Verification items for the finished model (mm, model axes). A direction names the side the tool comes from. Coordinates: 2 decimals unless noted, no trailing zeros. Loops run counter-clockwise (first coordinate to the right, second up) from the corner with the lowest first, then second, coordinate; pieces in that order, holes last.
Q1. Material ranges on probe 1 along X at (y, z) = (0, 9); probe 2 along Y at (x, z) = (0, -14.95); probe 3 along Z at (x, y) = (0, 13), recorded low to high.
Q2. Mould release check, pull along X, two halves, no side actions. Record for faces 4 (the face through (-0.1, -1.4, 6.6)), 5 (the face through (-2.548, -5.312, 12.573)), 6 (the face through (3, 36, -13.75)), 7 (the face through (-7.707, 29.632, -19.215)): +X half, -X half, draft (parallel to the pull), parting line (faces both ways), or undercut.
Q3. Sectioned sample at D-D (y = 17.5). Enter the section's corners in (x, z).
Q4. Go/stop test with flat-tipped pins: P1, Ø9, axis at y = 8.5, z = -9.5, coming from the +X side; P2, Ø6, axis at x = -6.5, y = 10.5, coming from the +Z side; P3, Ø5, axis at x = 6, z = -2, coming from the -Y side; P4, Ø3, axis at y = 24.5, z = -15.5, coming from the +X side. Record where each tip stops, or that it passes through.
Q5. Sectioned sample at C-C (x = 0). Count the separate pieces of the cut face and the enclosed holes in it, then the cut area to 3 significant figures.
Q6. Access from +Z, -Z, +X, -X, +Y, -Y to the whole of each face (thin tool, end or side, straight path). Record for faces 1 (the face through (0, 26, -16.75)), 2 (the face through (0, 2.5, 5)), 3 (the face through (-7.5, 2.7, -9.7)).
```python
from build123d import *

# Parameters (mm, degrees)
BOSS_EXTRUDE5_DEPTH      = 7.5
BOSS_EXTRUDE5_DEPTH_BACK = 7.5
SKETCH8_W                = 33.5
SKETCH8_H                = 5
SKETCH9_R                = 10
BOSS_EXTRUDE6_DEPTH      = 5
SKETCH11_R               = 2.65
CUT_EXTRUDE7_DEPTH       = 5
SKETCH12_R               = 4
SKETCH12_R_2             = 2.65
BOSS_EXTRUDE7_DEPTH      = 3
CHAMFER1_SIZE            = 3
FILLET1_R                = 10
FILLET2_R                = 5
SKETCH13_R               = 2.65
CUT_EXTRUDE8_DEPTH       = 50
SKETCH14_R               = 4
SKETCH14_R_2             = 2.65
BOSS_EXTRUDE8_DEPTH      = 3
CHAMFER2_SIZE            = 3


with BuildPart() as part:
    # Sketch8 → Boss-Extrude5 (new, two sides: drawn at the far end of the back side and taken through both)
    with BuildSketch(Plane.ZY.offset(-BOSS_EXTRUDE5_DEPTH_BACK)):
        Rectangle(SKETCH8_W, SKETCH8_H)
        Polygon((-16.75, -2.5), (-16.75, 2.5), (-16.75, 41.5), (-21.75, 41.5), (-21.75, -2.5), align=None)
    extrude(amount=BOSS_EXTRUDE5_DEPTH + BOSS_EXTRUDE5_DEPTH_BACK)

    # Sketch9 → Boss-Extrude6 (add)
    with BuildSketch(Plane.XY.offset(-16.75)):
        with Locations((0, 36.5)):
            Circle(SKETCH9_R)
    extrude(amount=-BOSS_EXTRUDE6_DEPTH)

    # Sketch11 → Cut-Extrude7 (cut)
    with BuildSketch(Plane(origin=(0, 0, -21.75), x_dir=(-1, 0, 0), z_dir=(0, 0, -1))):
        with Locations((0, 36.5)):
            Circle(SKETCH11_R)
    extrude(amount=-CUT_EXTRUDE7_DEPTH, mode=Mode.SUBTRACT)

    # Sketch12 → Boss-Extrude7 (add)
    with BuildSketch(Plane.XY.offset(-16.75)):
        with Locations((0, 36.5)):
            Circle(SKETCH12_R)
        with Locations(Location((0, 36.5, 0), (0, 0, 180))):
            Circle(SKETCH12_R_2, mode=Mode.SUBTRACT)
    extrude(amount=BOSS_EXTRUDE7_DEPTH)

    # Chamfer1
    chamfer1_edges = [part.edges().sort_by_distance(p)[0] for p in [
        (-4, 36.5, -16.75),
    ]]
    chamfer(chamfer1_edges, length=CHAMFER1_SIZE - 0.0001)  # a hair under: the kernel refuses the full size

    # Fillet1
    fillet1_edges = [part.edges().sort_by_distance(p)[0] for p in [
        (0, -2.5, -21.75),
        (0, 2.5, -16.75),
    ]]
    fillet(fillet1_edges, radius=FILLET1_R)

    # Fillet2
    fillet2_edges = [part.edges().sort_by_distance(p)[0] for p in [
        (-7.5, 29.885621722, -19.25),
        (7.5, 29.885621722, -19.25),
    ]]
    fillet(fillet2_edges, radius=FILLET2_R)

    # Sketch13 → Cut-Extrude8 (cut)
    with BuildSketch(Plane(origin=(0, 2.5, 0), x_dir=(1, 0, 0), z_dir=(0, 1, 0))):
        with Locations(Location((0, -9.25, 0), (0, 0, 270))):
            Circle(SKETCH13_R)
    extrude(amount=-CUT_EXTRUDE8_DEPTH, mode=Mode.SUBTRACT)

    # Sketch14 → Boss-Extrude8 (add)
    with BuildSketch(Plane.XZ.offset(2.5)):
        with Locations(Location((0, 9.25, 0), (0, 0, 270))):
            Circle(SKETCH14_R)
        with Locations(Location((0, 9.25, 0), (0, 0, 90))):
            Circle(SKETCH14_R_2, mode=Mode.SUBTRACT)
    extrude(amount=BOSS_EXTRUDE8_DEPTH)

    # Chamfer2
    chamfer2_edges = [part.edges().sort_by_distance(p)[0] for p in [
        (0, -2.5, 13.25),
    ]]
    chamfer(chamfer2_edges, length=CHAMFER2_SIZE - 0.0001)  # a hair under: the kernel refuses the full size


solid = part.part
```
Geometry check:
1. probe 1: x = -7.5 to -2.64, 2.64 to 7.5
1. probe 2: y = -1.97 to 6.78, 31.3 to 33.85, 39.15 to 41.7
1. probe 3: z = -21.75 to -16.75
2. face 4: undercut
2. face 5: parting line
2. face 6: draft
2. face 7: -X half
3. outline: (-7.5, -21.75) - (7.5, -21.75) - (7.5, -16.75) - (-7.5, -16.75) - close
4. P1: passes through
4. P2: stops at z = -15.41
4. P3: stops at y = -2.5
4. P4: stops at x = 7.5
5. separate pieces: 3
5. enclosed holes: 0
5. area: 394 mm2
6. face 1: +Z
6. face 2: +Z, +X, -X, +Y
6. face 3: +Z, -Z, -X, -Y
